Design review of the part built by this model. Coordinates are the model's own, in mm. A direction names the side the tool comes from. Coordinates: 2 decimals unless noted, no trailing zeros. Write each loop counter-clockwise with the first axis right and the second up, starting at its lowest first coordinate (ties: lowest second). Pieces come first, ordered by that corner, then holes. Notation, with made-up numbers: (51.5, -35.5) -> (58.5, -35.5) arc R19 cw to (58.5, -31.5) -> close; hole circle Ø4 at (46.5, 45). An arc over 180 degrees is marked (long way). Answer in a Markdown table with one row per item. Add a question column.
Item 1: Take a section at A-A, the plane x = 0. Write out the cut boundary in (y, z), and give its area (3 significant figures).
Item 2: Draft analysis for pull direction Z (two halves, no side actions). For faces 3 (the face through (4.132, 0.844, -0.543)), 4 (the face through (0.751, -0.424, 2.385)), 5 (the face through (-2, 1.266, 2)), state which applies: released by +Z, released by -Z, zero draft, split by the parting line, or undercut.
Item 3: Take a section at C-C, the plane y = 0.1. Write out the cut boundary in (x, z).
Item 4: Take a section at D-D, the plane x = -3.5. Write out the cut boundary in (y, z), and give its area (3 significant figures).
Item 5: For faces 1 (the face through (-6.1, -0.8, -1.36)), 2 (the face through (-4.1, 0.433, -1.5)), list the 3-axis set-ups (+Z, -Z, +X, -X, +Y, -Y) from which the entire face can be reached by the end or side of a thin tool; tool diameter is ignored.
Item 6: Take a section at B-B, the plane z = 0. Write out the cut boundary in (x, y).
Item 7: To check wall thickness, follow line 1 (X direction, y = -0.6, z = 0); line 2 (X direction, y = 0.5, z = 0); line 3 (Z direction, x = -2.25, y = -0.5). State the ranges of each line that lie inside material, in increasing order.
Item 8: Clearance check with a flat-ended pin moving along its axis: P1, Ø1, axis at y = 0, z = 1, coming from the -X side. State where the tip first meets the part, or that it passes through.
from build123d import *

# Parameters (mm, degrees)
SKETCH1_R           = 3.75
SKETCH1_R_2         = 2.5
SKETCH1_R_3         = 1.5
BOSS_EXTRUDE1_DEPTH = 1.5
SKETCH1_3_R         = 2.5
SKETCH1_3_R_2       = 1.5
BOSS_EXTRUDE2_DEPTH = 0.5
SCALE1_SCALE        = 1.667


with BuildPart() as part:
    # Sketch1 → Boss-Extrude1 (new body)
    with BuildSketch(Plane(origin=(0, 0, 0), x_dir=(1, 0, 0), z_dir=(0, 1, 0))):
        with Locations(Location((0, 0, 0), (0, 0, 270))):
            Circle(SKETCH1_R)
        Circle(SKETCH1_R_2, mode=Mode.SUBTRACT)
        Circle(SKETCH1_R_2)
        with Locations(Location((0, 0, 0), (0, 0, 270))):
            Circle(SKETCH1_R_3, mode=Mode.SUBTRACT)
    extrude(amount=-BOSS_EXTRUDE1_DEPTH)

    # Sketch1_3 → Boss-Extrude2 (add)
    with BuildSketch(Plane(origin=(0, 0, 0), x_dir=(1, 0, 0), z_dir=(0, 1, 0))):
        with Locations(Location((0, 0, 0), (0, 0, 270))):
            Circle(SKETCH1_3_R)
        with Locations(Location((0, 0, 0), (0, 0, 270))):
            Circle(SKETCH1_3_R_2, mode=Mode.SUBTRACT)
    extrude(amount=BOSS_EXTRUDE2_DEPTH)


with BuildPart() as part_1:
    # Scale1: scaled about (0, -0.648573693, 0)
    add(part.part.scale(SCALE1_SCALE).moved(Location((0, 0.432598653, 0))))


solid = part_1.part
Answers:
| question | item | result |
|---|---|---|
| 1 | outline | (-2.07, -6.25) -> (0.43, -6.25) -> (0.43, -4.17) -> (1.27, -4.17) -> (1.27, -2.5) -> (-2.07, -2.5) -> close; (-2.07, 2.5) -> (1.27, 2.5) -> (1.27, 4.17) -> (0.43, 4.17) -> (0.43, 6.25) -> (-2.07, 6.25) -> close |
| 1 | area | 21.5 mm^2 |
| 2 | face 3 | split by the parting line |
| 2 | face 4 | undercut |
| 2 | face 5 | zero draft |
| 3 | outline | circle Ø12.5 at (0, 0); hole circle Ø5 at (0, 0) |
| 4 | outline | (-2.07, -5.18) -> (0.43, -5.18) -> (0.43, -2.26) -> (1.27, -2.26) -> (1.27, 2.26) -> (0.43, 2.26) -> (0.43, 5.18) -> (-2.07, 5.18) -> close |
| 4 | area | 29.7 mm^2 |
| 5 | face 1 | +Y, -Y |
| 5 | face 2 | +Y |
| 6 | outline | (-6.25, -2.07) -> (-2.5, -2.07) -> (-2.5, 1.27) -> (-4.17, 1.27) -> (-4.17, 0.43) -> (-6.25, 0.43) -> close; (2.5, -2.07) -> (6.25, -2.07) -> (6.25, 0.43) -> (4.17, 0.43) -> (4.17, 1.27) -> (2.5, 1.27) -> close |
| 7 | line 1 | x = -6.25 to -2.5, 2.5 to 6.25 |
| 7 | line 2 | x = -4.17 to -2.5, 2.5 to 4.17 |
| 7 | line 3 | z = -5.83 to -1.09, 1.09 to 5.83 |
| 8 | P1 | stops at x = -6.23 |
